Could you check a few things on this drawing? It's one solid part, dimensions in mm from its lowest x, y, z. A direction names the side the tool comes from. Give positions to 0.01 mm unless a question says otherwise; leave off trailing zeros. Write each loop counter-clockwise with the first axis right and the second up, starting at its lowest first coordinate (ties: lowest second). Pieces come first, ordered by that corner, then holes. Notation, with made-up numbers: M 13,-14 L 17,-14 A16 cw 17,-1 Z; hole C 3.25,77 d8. An arc over 180 degrees is marked long. Write each question's results on one line, items separated by ' | '.
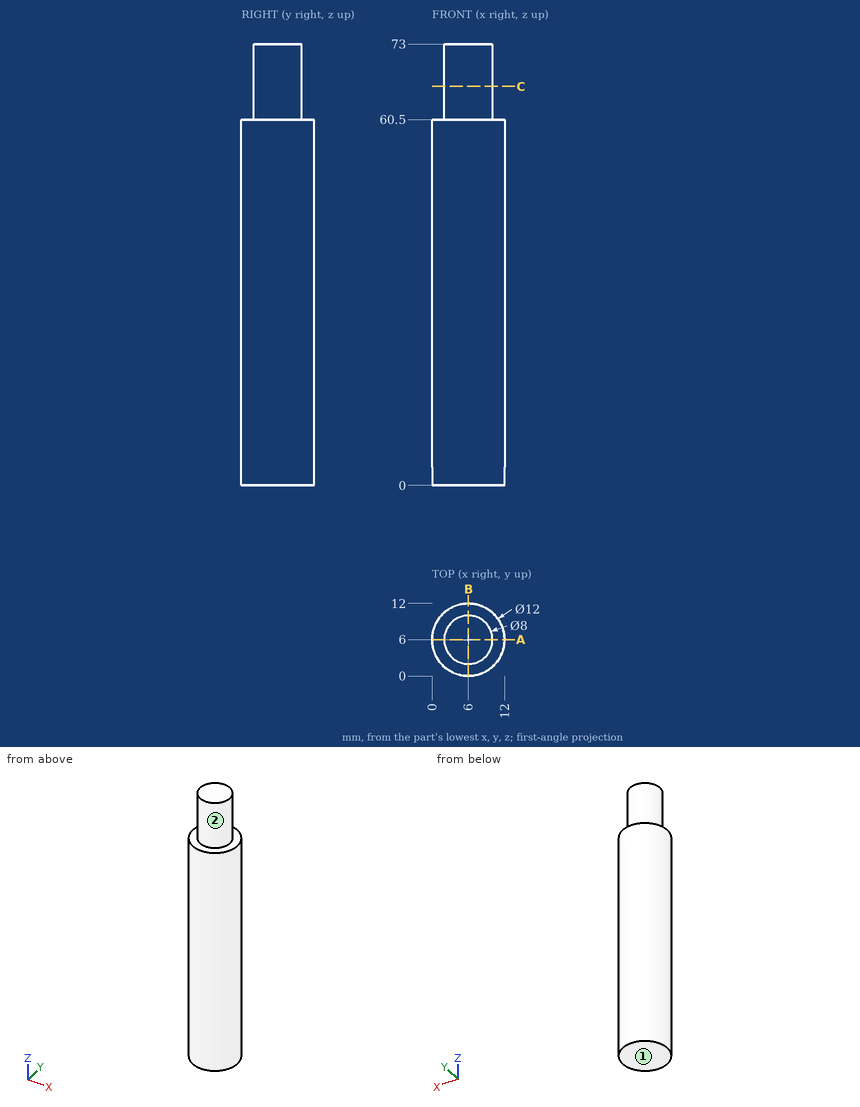
Item 1: I'm going to push a flat-ended pin straight in: pin 1 (5 mm diameter, centred on x = 2, z = 13.5, fed in from -Y). Where does the tip first touch, or does it pass through?
Geometry says:
pin 1: stops at y = 0.19
Item 2: I want a section at A-A, the plane y = 6. Please give me the cut outline in (x, z).
Geometry says:
outline: M 0,0 L 12,0 L 12,60.5 L 10,60.5 L 10,73 L 2,73 L 2,60.5 L 0,60.5 Z
Item 3: If I drill on line 1 (Y direction, x = 6.25, z = 67); line 2 (Z direction, x = 4.25, y = 1.25); line 3 (Y direction, x = 4, z = 43), over which ranges is the centre line in solid material (lowest first)? Write a range as from..to.
Geometry says:
line 1: y = 2.01..9.99 | line 2: z = 0..60.5 | line 3: y = 0.34..11.66
Item 4: For the marked faces 1 and 2, which set-ups out of +Z, -Z, +X, -X, +Y, -Y let a thin tool reach every point of the face, with its end or its side?
Geometry says:
face 1: -Z, +X, -X, +Y, -Y | face 2: +Z
Item 5: I want a section at C-C, the plane z = 66. Please give me the cut outline in (x, y).
Geometry says:
outline: C 6,6 d8
